Study the drawing (mm; zero at the part's minimum x, y, z) and answer. Coordinates: 2 decimals unless noted, no trailing zeros. Order: outer loops, then holes, each group sorted by start corner. A loop starts at its lowest first (then second) coordinate and runs counter-clockwise, first axis right, second up.
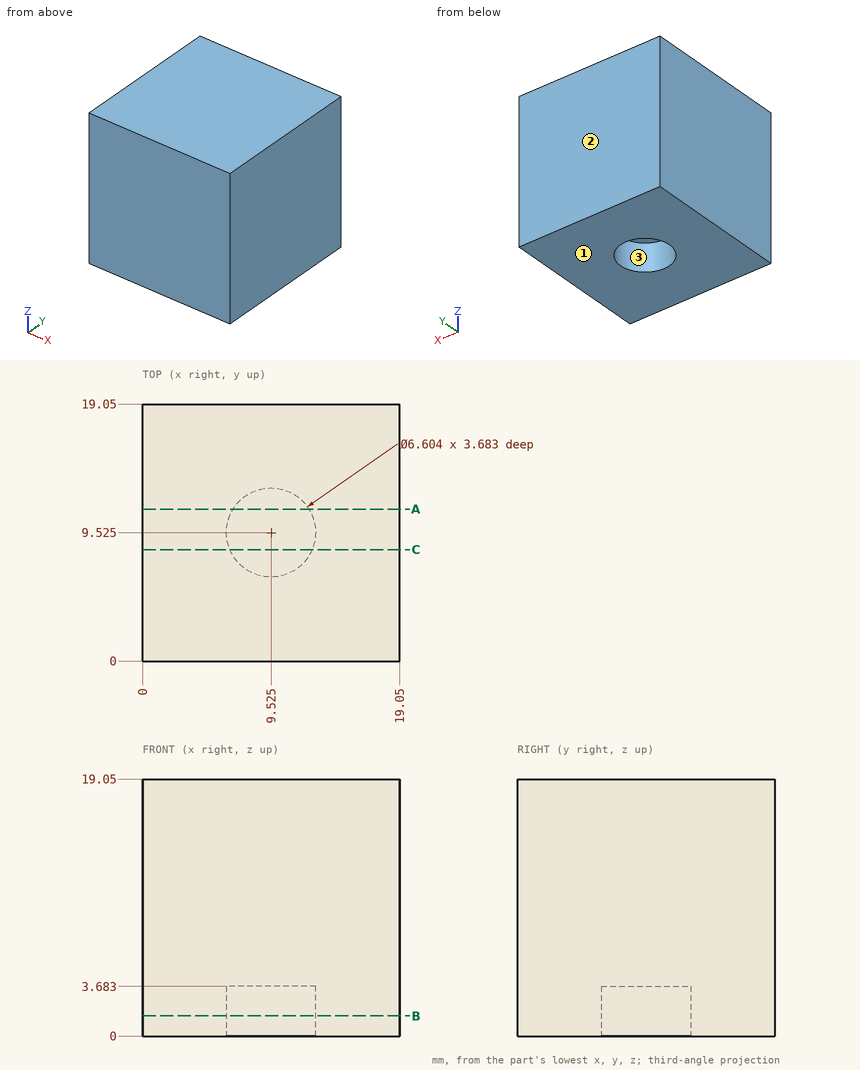
1) Determine the mould class of the marked faces 1, 2 and 3 for opening direction Y: pulls with the +Y half, pulls with the -Y half, needs draft (parallel to the pull), parting line crosses it, or undercut.
A:
face 1: needs draft
face 2: pulls with the +Y half
face 3: undercut
2) A cutting plane is placed at A-A, the plane y = 11.25. Determine the outline of the cut face in (x, z), and give its area (3 significant figures).
A:
outline: (0, 0) - (6.71, 0) - (6.71, 3.68) - (12.34, 3.68) - (12.34, 0) - (19.05, 0) - (19.05, 19.05) - (0, 19.05) - close
area: 342 mm2
3) Straight lines are drawn through the part: line 1 (Y direction, x = 7.75, z = 1.75); line 2 (Y direction, x = 12, z = 2.25). For each, find the intervals that lie inside material, in ascending order.
A:
line 1: y = 0 to 6.74, 12.31 to 19.05
line 2: y = 0 to 7.34, 11.71 to 19.05
4) A cutting plane is placed at C-C, the plane y = 8.25. Determine the outline of the cut face in (x, z), and give its area (3 significant figures).
A:
outline: (0, 0) - (6.48, 0) - (6.48, 3.68) - (12.57, 3.68) - (12.57, 0) - (19.05, 0) - (19.05, 19.05) - (0, 19.05) - close
area: 340 mm2
5) A cutting plane is placed at B-B, the plane z = 1.5. Determine the outline of the cut face in (x, y) (3 decimals).
A:
outline: (0, 0) - (19.05, 0) - (19.05, 19.05) - (0, 19.05) - close; hole circle Ø6.604 at (9.525, 9.525)
